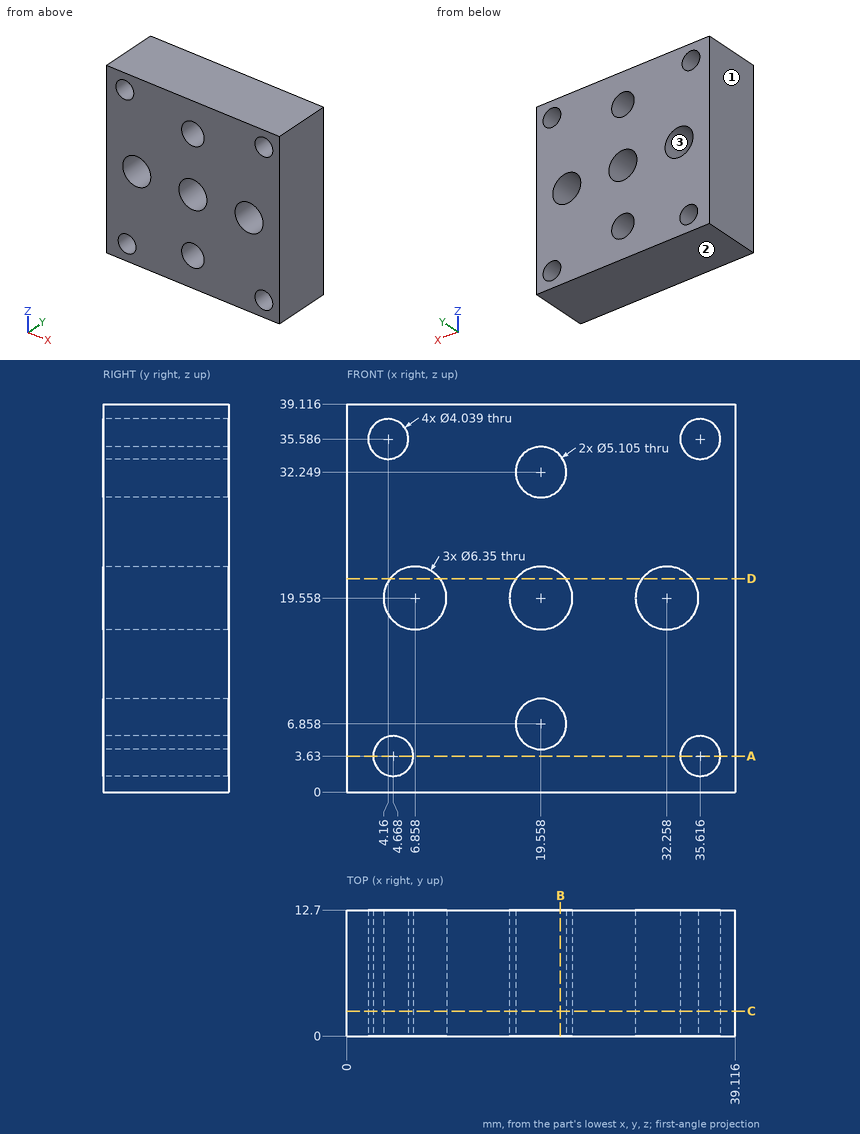
Here's the drawing with two shaded views (mm, measured from the low corner). I have some questions. Give positions to 0.01 mm unless a question says otherwise; leave off trailing zeros. Order: outer loops, then holes, each group sorted by start corner. A loop starts at its lowest first (then second) coordinate and runs counter-clockwise, first axis right, second up. Notation, with made-up numbers: (-8, 15) -> (16, 15) arc R20 ccw to (16, 19) -> close; hole circle Ø5 at (24, 29). An arc over 180 degrees is marked (long way). One line per item, written item: value. Start each with the question number.
1. Will these pins go through, and if not, where does the flat tip stop? pin 1 Ø8 at (x, z) = (34.5, 25.5) entering from -Y; pin 2 Ø3.5 at (x, z) = (35.616, 3.63) entering from +Y.
2. Imagine slicing it at A-A, the plane z = 3.63. List the corners of the cut face in (x, y) for me (1 decimal), plus the area to 3 significant figures.
3. Imagine slicing it at C-C, the plane y = 2.5. Count the separate pieces of the cut face and the enclosed holes in it, plus the area to 3 significant figures.
4. We'd pull the mould along Z, two halves only. Please class the marked faces 1, 2 and 3: released by +Z, released by -Z, zero draft, split by the parting line, or undercut.
5. Imagine slicing it at D-D, the plane z = 21.5. List the corners of the cut face in (x, y) for me, plus the area to 3 significant figures.
6. I need wall thicknesses on probe 1 along X at (y, z) = (9, 3.63) (1 decimal); probe 2 along Z at (x, y) = (4.16, 9.5) (1 decimal); probe 3 along X at (y, z) = (9.75, 17.5) (1 decimal). Which ranges of each line are inside material? Lowest first, please. Write a range as from..to.
7. Imagine slicing it at B-B, the plane x = 21.5. List the corners of the cut face in (y, z) for me (1 decimal).
Values follow:
1. pin 1: stops at y = 0
1. pin 2: passes through
2. outline: (0, 0) -> (2.6, 0) -> (2.6, 12.7) -> (0, 12.7) -> close; (6.7, 0) -> (33.6, 0) -> (33.6, 12.7) -> (6.7, 12.7) -> close; (37.6, 0) -> (39.1, 0) -> (39.1, 12.7) -> (37.6, 12.7) -> close
2. area: 394 mm2
3. separate pieces: 1
3. enclosed holes: 9
3. area: 1,340 mm2
4. face 1: zero draft
4. face 2: released by -Z
4. face 3: undercut
5. outline: (0, 0) -> (4.35, 0) -> (4.35, 12.7) -> (0, 12.7) -> close; (9.37, 0) -> (17.05, 0) -> (17.05, 12.7) -> (9.37, 12.7) -> close; (22.07, 0) -> (29.75, 0) -> (29.75, 12.7) -> (22.07, 12.7) -> close; (34.77, 0) -> (39.12, 0) -> (39.12, 12.7) -> (34.77, 12.7) -> close
5. area: 305 mm2
6. probe 1: x = 0..2.6, 6.7..33.6, 37.6..39.1
6. probe 2: z = 0..1.7, 5.6..17.9, 21.2..33.6, 37.6..39.1
6. probe 3: x = 0..4.4, 9.3..17.1, 22..29.8, 34.7..39.1
7. outline: (0, 0) -> (12.7, 0) -> (12.7, 5.2) -> (0, 5.2) -> close; (0, 8.5) -> (12.7, 8.5) -> (12.7, 17) -> (0, 17) -> close; (0, 22.1) -> (12.7, 22.1) -> (12.7, 30.6) -> (0, 30.6) -> close; (0, 33.9) -> (12.7, 33.9) -> (12.7, 39.1) -> (0, 39.1) -> close
